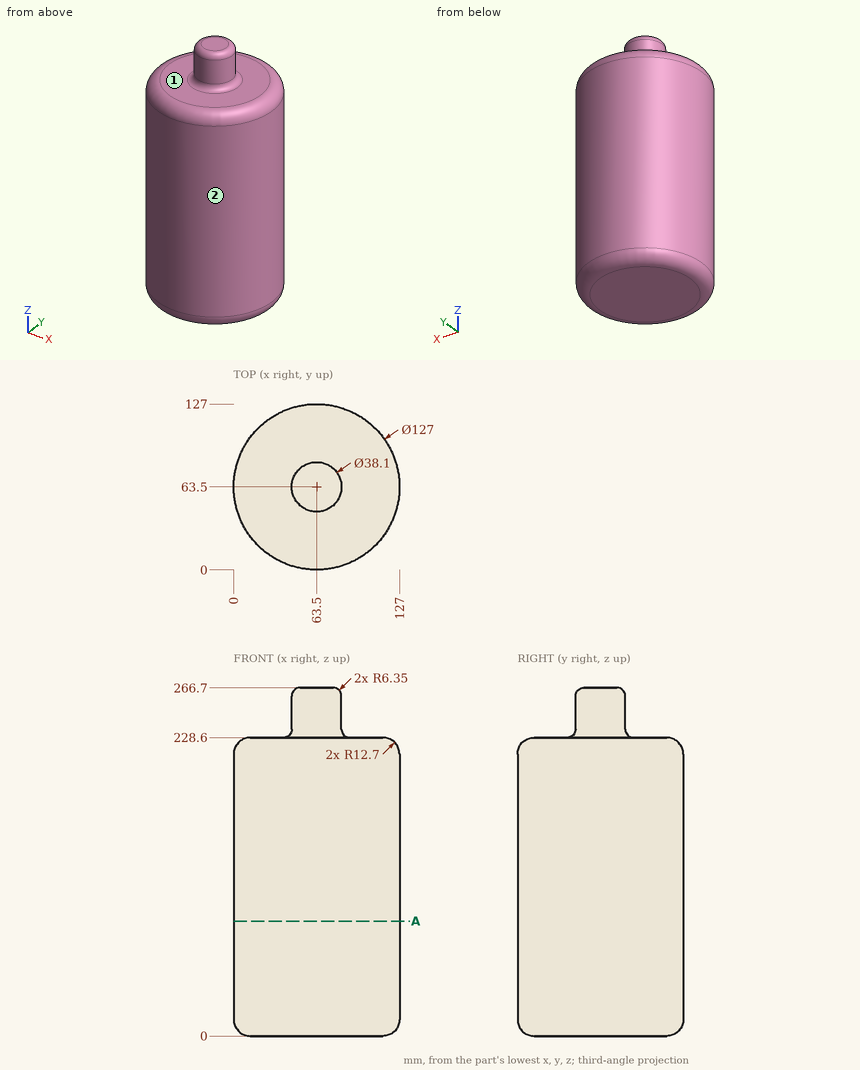
Study the drawing (mm; zero at the part's minimum x, y, z) and answer. A direction names the side the tool comes from. Give positions to 0.01 mm unless a question says otherwise; leave off trailing zeros. Loops run counter-clockwise (first coordinate to the right, second up) from the corner with the lowest first, then second, coordinate; pieces in that order, holes last. Notation, with made-up numbers: (13.5, 7.25) -> (41.5, 7.25) arc R32 ccw to (41.5, 40.25) -> close; hole circle Ø9 at (-22.75, -22.75). An arc over 180 degrees is marked (long way). Use a Markdown table: item, result. Add a question column.
1) Which of the six approach directions +Z, -Z, +X, -X, +Y, -Y give full straight-line access (tool end or side, diameter ignored) to the marked faces 1 and 2?
2) Consider line 1 along Z through (x, y) = (73.5, 97); line 2 along X through (y, z) = (64, 235.5); line 3 along Y through (x, z) = (15.5, 143.5). Determine where each line is inside the solid, lowest interval first.
3) Each of these flat-tipped pins is pushed along its axis until it touches: P1, Ø1, axis at x = 55.5, y = 63, coming from the -Z side; P2, Ø2, axis at x = 15, y = 76.5, coming from the +Z side; P3, Ø6, axis at x = 98.5, y = 15, coming from the +Z side; P4, Ø8, axis at x = 108, z = 178.5, coming from the +Y side. Where does it stop, or does it pass through?
4) The part is cut by section A-A, the plane z = 88. Determine the outline of the cut face in (x, y), plus the area to 3 significant figures.
Reported:
| question | item | result |
|---|---|---|
| 1 | face 1 | +Z |
| 1 | face 2 | +Z, -Z |
| 2 | line 1 | z = 0 to 228.6 |
| 2 | line 2 | x = 44.46 to 82.54 |
| 2 | line 3 | y = 21.93 to 105.07 |
| 3 | P1 | stops at z = 0 |
| 3 | P2 | stops at z = 228.6 |
| 3 | P3 | stops at z = 227.09 |
| 3 | P4 | stops at y = 112.41 |
| 4 | outline | circle Ø127 at (63.5, 63.5) |
| 4 | area | 12,700 mm^2 |
